from build123d import *

# Parameters (mm, degrees)
SKETCH1_W               = 70
SKETCH1_H               = 80
BOSS_EXTRUDE1_DEPTH     = 21.5
FILLET1_R               = 5
SHELL1_T                = 3
BOSS_EXTRUDE2_REACH     = 59.335
SKETCH3_R               = 5
SPLIT2_SURFACE_1_BACK   = 109.454
SPLIT2_SURFACE_1_DEPTH  = 218.908
SPLIT2_SURFACE_2_BACK   = 109.454
SPLIT2_SURFACE_2_DEPTH  = 218.908
SKETCH4_R               = 1
CUT_EXTRUDE1_DEPTH      = 58.334544561
SKETCH5_R               = 3
CUT_EXTRUDE2_DEPTH      = 7.75
SKETCH6_OUTSIDE_W       = 93.69
SKETCH6_OUTSIDE_H       = 103.69
CUT_EXTRUDE3_DEPTH      = 2
BOSS_EXTRUDE3_START     = 1.7
BOSS_EXTRUDE3_DEPTH     = 1.7
SKETCH8_R               = 5.5
CUT_EXTRUDE4_DEPTH      = 10
SKETCH9_R               = 5
SKETCH9_W               = 20
SKETCH9_H               = 12
CUT_EXTRUDE5_DEPTH      = 10
BOSS_EXTRUDE4_OUTLINE_W = 20
BOSS_EXTRUDE4_OUTLINE_H = 1.5
BOSS_EXTRUDE4_DEPTH     = 7.75
SKETCH12_W              = 29.5
SKETCH12_H              = 12
CUT_EXTRUDE6_DEPTH      = 10
BOSS_EXTRUDE5_DEPTH     = 5


# Read off the part's stored shape, not the designer's step: Boss-Extrude4
with BuildPart() as part:
    # Sketch1 → Boss-Extrude1 (new body)
    with BuildSketch(Plane(origin=(0, 0, 0), x_dir=(1, 0, 0), z_dir=(0, 1, 0))):
        Rectangle(SKETCH1_W, SKETCH1_H)
    extrude(amount=BOSS_EXTRUDE1_DEPTH)

    # Fillet1
    fillet1_edges = [part.edges().sort_by_distance(p)[0] for p in [
        (-35, 10.75, -40),
        (35, 10.75, -40),
        (35, 10.75, 40),
        (-35, 10.75, 40),
    ]]
    fillet(fillet1_edges, radius=FILLET1_R)

    # Shell1 (no face opened: a closed hollow body)
    add(offset(amount=-SHELL1_T, mode=Mode.PRIVATE), mode=Mode.SUBTRACT)

    # Sketch3 → Boss-Extrude2 (add, up to next)
    with BuildSketch(Plane(origin=(0, 21.5, 0), x_dir=(1, 0, 0), z_dir=(0, 1, 0)), mode=Mode.PRIVATE) as boss_extrude2_sk1:
        with Locations((-30, 35)):
            Circle(SKETCH3_R)
    boss_extrude2_tool1 = extrude(boss_extrude2_sk1.sketch, amount=-BOSS_EXTRUDE2_REACH, mode=Mode.PRIVATE) - part.part
    # Sketch3 → Boss-Extrude2 (add, up to next)
    with BuildSketch(Plane(origin=(0, 21.5, 0), x_dir=(1, 0, 0), z_dir=(0, 1, 0)), mode=Mode.PRIVATE) as boss_extrude2_sk2:
        with Locations((30, 35)):
            Circle(SKETCH3_R)
    boss_extrude2_tool2 = extrude(boss_extrude2_sk2.sketch, amount=-BOSS_EXTRUDE2_REACH, mode=Mode.PRIVATE) - part.part
    # Sketch3 → Boss-Extrude2 (add, up to next)
    with BuildSketch(Plane(origin=(0, 21.5, 0), x_dir=(1, 0, 0), z_dir=(0, 1, 0)), mode=Mode.PRIVATE) as boss_extrude2_sk3:
        with Locations((30, -35)):
            Circle(SKETCH3_R)
    boss_extrude2_tool3 = extrude(boss_extrude2_sk3.sketch, amount=-BOSS_EXTRUDE2_REACH, mode=Mode.PRIVATE) - part.part
    # Sketch3 → Boss-Extrude2 (add, up to next)
    with BuildSketch(Plane(origin=(0, 21.5, 0), x_dir=(1, 0, 0), z_dir=(0, 1, 0)), mode=Mode.PRIVATE) as boss_extrude2_sk4:
        with Locations((-30, -35)):
            Circle(SKETCH3_R)
    boss_extrude2_tool4 = extrude(boss_extrude2_sk4.sketch, amount=-BOSS_EXTRUDE2_REACH, mode=Mode.PRIVATE) - part.part
    add(boss_extrude2_tool1.solids().sort_by_distance((-30, 21.5, -35))[0])
    add(boss_extrude2_tool2.solids().sort_by_distance((30, 21.5, -35))[0])
    add(boss_extrude2_tool3.solids().sort_by_distance((30, 21.5, 35))[0])
    add(boss_extrude2_tool4.solids().sort_by_distance((-30, 21.5, 35))[0])


with BuildPart() as body_2:
    # Split2: the piece behind the surface
    add(part.part)
    # Split2 surface: a surface, the sketch's curves swept straight by 218.908 mm
    with BuildLine(Plane(origin=(0, 0, 0), x_dir=(0, 0, -1), z_dir=(1, 0, 0)).offset(-SPLIT2_SURFACE_1_BACK), mode=Mode.PRIVATE) as split2_surface_1_path:
        Line((-40, 10.75), (51.562362236, 10.75))
    split2_surface_1 = Shell.extrude(split2_surface_1_path.wire(), (1 * SPLIT2_SURFACE_1_DEPTH, 0 * SPLIT2_SURFACE_1_DEPTH, 0 * SPLIT2_SURFACE_1_DEPTH))
    split(bisect_by=split2_surface_1, keep=Keep.BOTTOM)


with BuildPart() as part_1:
    add(part.part)

    # Split2: split by a surface, the side it looks to stays
    # Split2 surface: a surface, the sketch's curves swept straight by 218.908 mm
    with BuildLine(Plane(origin=(0, 0, 0), x_dir=(0, 0, -1), z_dir=(1, 0, 0)).offset(-SPLIT2_SURFACE_2_BACK), mode=Mode.PRIVATE) as split2_surface_2_path:
        Line((-40, 10.75), (51.562362236, 10.75))
    split2_surface_2 = Shell.extrude(split2_surface_2_path.wire(), (1 * SPLIT2_SURFACE_2_DEPTH, 0 * SPLIT2_SURFACE_2_DEPTH, 0 * SPLIT2_SURFACE_2_DEPTH))
    split(bisect_by=split2_surface_2, keep=Keep.TOP)


with BuildPart() as cut_extrude1_tool:
    # Sketch4 → Cut-Extrude1 (new, through all)
    with BuildSketch(Plane(origin=(0, 21.5, 0), x_dir=(1, 0, 0), z_dir=(0, 1, 0))):
        with Locations(Location((-30, 35, 0), (0, 0, 270))):
            Circle(SKETCH4_R)
        with Locations(Location((30, 35, 0), (0, 0, 270))):
            Circle(SKETCH4_R)
        with Locations(Location((30, -35, 0), (0, 0, 270))):
            Circle(SKETCH4_R)
        with Locations(Location((-30, -35, 0), (0, 0, 270))):
            Circle(SKETCH4_R)
    extrude(amount=-CUT_EXTRUDE1_DEPTH)


with BuildPart() as part_2:
    add(part_1.part)

    # Cut-Extrude1: cut by cut_extrude1_tool
    add(cut_extrude1_tool.part, mode=Mode.SUBTRACT)

    # Sketch5 → Cut-Extrude2 (cut)
    with BuildSketch(Plane(origin=(0, 21.5, 0), x_dir=(1, 0, 0), z_dir=(0, 1, 0))):
        with Locations(Location((-30, 35, 0), (0, 0, 270))):
            Circle(SKETCH5_R)
        with Locations(Location((30, 35, 0), (0, 0, 270))):
            Circle(SKETCH5_R)
        with Locations(Location((30, -35, 0), (0, 0, 270))):
            Circle(SKETCH5_R)
        with Locations(Location((-30, -35, 0), (0, 0, 270))):
            Circle(SKETCH5_R)
    extrude(amount=-CUT_EXTRUDE2_DEPTH, mode=Mode.SUBTRACT)

    # Sketch6 outside → Cut-Extrude3 (cut)
    with BuildSketch(Plane.XZ.offset(-10.75)):
        Rectangle(SKETCH6_OUTSIDE_W, SKETCH6_OUTSIDE_H)
        with BuildLine():
            Line((-30, -38.5), (30, -38.5))
            ThreePointArc((30, -38.5), (32.474873734, -37.474873734), (33.5, -35))
            Line((33.5, -35), (33.5, 35))
            ThreePointArc((33.5, 35), (32.474873734, 37.474873734), (30, 38.5))
            Line((30, 38.5), (-30, 38.5))
            ThreePointArc((-30, 38.5), (-32.474873734, 37.474873734), (-33.5, 35))
            Line((-33.5, 35), (-33.5, -35))
            ThreePointArc((-33.5, -35), (-32.474873734, -37.474873734), (-30, -38.5))
        make_face(mode=Mode.SUBTRACT)
    extrude(amount=-CUT_EXTRUDE3_DEPTH, mode=Mode.SUBTRACT)


with BuildPart() as body_2_1:
    add(body_2.part)

    # Cut-Extrude1: cut by cut_extrude1_tool
    add(cut_extrude1_tool.part, mode=Mode.SUBTRACT)

    # Sketch7 → Boss-Extrude3 (add)
    with BuildSketch(Plane(origin=(0, 10.75, 0), x_dir=(1, 0, 0), z_dir=(0, 1, 0)).offset(BOSS_EXTRUDE3_START)):
        with BuildLine():
            Line((-30, 40), (30, 40))
            ThreePointArc((30, 40), (33.535533906, 38.535533906), (35, 35))
            Line((35, 35), (35, -35))
            ThreePointArc((35, -35), (33.535533906, -38.535533906), (30, -40))
            Line((30, -40), (-30, -40))
            ThreePointArc((-30, -40), (-33.535533906, -38.535533906), (-35, -35))
            Line((-35, -35), (-35, 35))
            ThreePointArc((-35, 35), (-33.535533906, 38.535533906), (-30, 40))
        make_face()
        with BuildLine():
            Line((30, 38.7), (-30, 38.7))
            ThreePointArc((-30, 38.7), (-32.61629509, 37.61629509), (-33.7, 35))
            Line((-33.7, 35), (-33.7, -35))
            ThreePointArc((-33.7, -35), (-32.61629509, -37.61629509), (-30, -38.7))
            Line((-30, -38.7), (30, -38.7))
            ThreePointArc((30, -38.7), (32.61629509, -37.61629509), (33.7, -35))
            Line((33.7, -35), (33.7, 35))
            ThreePointArc((33.7, 35), (32.61629509, 37.61629509), (30, 38.7))
        make_face(mode=Mode.SUBTRACT)
    extrude(amount=-BOSS_EXTRUDE3_DEPTH)


with BuildPart() as cut_extrude4_tool:
    # Sketch8 → Cut-Extrude4 (new body)
    with BuildSketch(Plane.ZY.offset(35)):
        with Locations((-20, 11.95)):
            Circle(SKETCH8_R)
    extrude(amount=-CUT_EXTRUDE4_DEPTH)


with BuildPart() as part_3:
    add(part_2.part)

    # Cut-Extrude4: cut by cut_extrude4_tool
    add(cut_extrude4_tool.part, mode=Mode.SUBTRACT)


with BuildPart() as body_2_2:
    add(body_2_1.part)

    # Cut-Extrude4: cut by cut_extrude4_tool
    add(cut_extrude4_tool.part, mode=Mode.SUBTRACT)


with BuildPart() as cut_extrude5_tool:
    # Sketch9 → Cut-Extrude5 (new body)
    with BuildSketch(Plane.XY.offset(40)):
        with Locations((16, 11.95)):
            Circle(SKETCH9_R)
        with Locations((-10, 10.75)):
            Rectangle(SKETCH9_W, SKETCH9_H)
    extrude(amount=-CUT_EXTRUDE5_DEPTH)


with BuildPart() as part_4:
    add(part_3.part)

    # Cut-Extrude5: cut by cut_extrude5_tool
    add(cut_extrude5_tool.part, mode=Mode.SUBTRACT)

    # Boss-Extrude4 outline → Boss-Extrude4 (add)
    with BuildSketch(Plane.XZ.offset(-18.5)):
        Polygon((10.5, 37), (7.5, 37), (7.5, 35), (6, 35), (6, 32), (10.5, 32), align=None)
        with Locations((-10, 37.75)):
            Rectangle(BOSS_EXTRUDE4_OUTLINE_W, BOSS_EXTRUDE4_OUTLINE_H)
        with BuildLine():
            Line((-23.5, 35), (-25, 35))
            ThreePointArc((-25, 35), (-25.25658351, 33.41886117), (-26, 32))
            Line((-26, 32), (-23.5, 32))
            Line((-23.5, 32), (-23.5, 35))
        make_face()
        with BuildLine():
            Line((-25, 35), (-25, 37))
            Line((-25, 37), (-25.417424305, 37))
            ThreePointArc((-25.417424305, 37), (-25.105468435, 36.021548218), (-25, 35))
        make_face()
        with BuildLine():
            Line((-28, 37.236067977), (-28, 32.763932023))
            ThreePointArc((-28, 32.763932023), (-27, 35), (-28, 37.236067977))
        make_face()
    extrude(amount=BOSS_EXTRUDE4_DEPTH)


with BuildPart() as body_2_3:
    add(body_2_2.part)

    # Cut-Extrude5: cut by cut_extrude5_tool
    add(cut_extrude5_tool.part, mode=Mode.SUBTRACT)


with BuildPart() as cut_extrude6_tool:
    # Sketch12 → Cut-Extrude6 (new body)
    with BuildSketch(Plane(origin=(0, 0, 37), x_dir=(-1, 0, 0), z_dir=(0, 0, -1))):
        with Locations((8.75, 10.75)):
            Rectangle(SKETCH12_W, SKETCH12_H)
    extrude(amount=-CUT_EXTRUDE6_DEPTH)


with BuildPart() as part_5:
    add(part_4.part)

    # Cut-Extrude6: cut by cut_extrude6_tool
    add(cut_extrude6_tool.part, mode=Mode.SUBTRACT)

    # Sketch14 → Boss-Extrude5 (add)
    with BuildSketch(Plane.XZ.offset(-10.75)):
        Polygon((10.5, 36.8), (7.5, 36.8), (7.5, 35), (6, 35), (6, 32), (10.5, 32), align=None)
    extrude(amount=BOSS_EXTRUDE5_DEPTH)


with BuildPart() as body_2_4:
    add(body_2_3.part)

    # Cut-Extrude6: cut by cut_extrude6_tool
    add(cut_extrude6_tool.part, mode=Mode.SUBTRACT)


solid = body_2_4.part
Verification items for the finished model (mm, model axes). A direction names the side the tool comes from. Give positions to 0.01 mm unless a question says otherwise; leave off trailing zeros. Loops run counter-clockwise (first coordinate to the right, second up) from the corner with the lowest first, then second, coordinate; pieces in that order, holes last. Notation, with made-up numbers: (55, -4.75) - (62, -4.75) arc R11 ccw to (62, 11.25) - close; hole circle Ø7 at (48.5, 18.5). An arc over 180 degrees is marked (long way). Write each question's results on one line, items separated by ' | '.
1) Sectioned sample at A-A on y = 8. Count the separate pieces of the cut face and the enclosed holes in it, plus the area to 3 significant figures.
Solution:
separate pieces: 3 | enclosed holes: 4 | area: 872 mm2
2) Material ranges on L1, parallel to X at y = 5.75, z = -35; L2, parallel to X at y = 4.25, z = -17; L3, parallel to Z at x = -1, y = 3.5, recorded low to high. Write a range as from..to.
Solution:
L1: -35..-31, -29..-25, 25..29, 31..35 | L2: -35..-32, 32..35 | L3: -40..-37, 37..40
3) Mould release check, pull along X, two halves, no side actions. Record for faces 1 (the flat face through (35, 6, 0)), 2 (the flat face through (32.3, 10.75, -14.2)), 3 (the flat face through (34, 12.45, -18)): pulls with the +X half, pulls with the -X half, needs draft (parallel to the pull), parting line crosses it, or undercut.
Solution:
face 1: pulls with the +X half | face 2: undercut | face 3: needs draft
4) Sectioned sample at B-B on x = 27. Record the boundary of the cut face in (y, z).
Solution:
outline: (0, -40) - (12.45, -40) - (12.45, -38.7) - (10.75, -38.7) - (10.75, -31) - (3, -31) - (3, 31) - (10.75, 31) - (10.75, 38.7) - (12.45, 38.7) - (12.45, 40) - (0, 40) - close
5) Tool access check on faces 4 (the flat face through (-9, 4.75, 38)), 5 (the flat face through (0, 7, -37)), 6 (the cylindrical face through (30.84, 5.45, -34.46)). Record the directions out of +Z, -Z, +X, -X, +Y, -Y that give a thin tool (end or side, any length) a straight path to the whole face; none if there is none.
Solution:
face 4: +Z, +Y | face 5: +Y | face 6: +Y, -Y
6) Depth check by flat-ended pin: P1, Ø8, axis at x = -10, z = 12, coming from the +Y side; P2, Ø2.5, axis at x = -30, z = -35, coming from the +Y side; P3, Ø4, axis at x = 6.5, z = -31, coming from the -Y side; P4, Ø1.5, axis at x = -2, z = 39, coming from the +Y side. Enter the tip coordinate at first touch or a pass-through.
Solution:
P1: y = 3 | P2: y = 10.75 | P3: y = 0 | P4: y = 4.75
7) Sectioned sample at C-C on z = -12. Record the boundary of the cut face in (x, y).
Solution:
outline: (-35, 0) - (35, 0) - (35, 12.45) - (33.7, 12.45) - (33.7, 10.75) - (32, 10.75) - (32, 3) - (-32, 3) - (-32, 10.75) - (-33.7, 10.75) - (-33.7, 12.45) - (-35, 12.45) - close
8) Sectioned sample at D-D on x = 16. Record the boundary of the cut face in (y, z), plus the area to 3 significant figures.
Solution:
outline: (0, -40) - (12.45, -40) - (12.45, -38.7) - (10.75, -38.7) - (10.75, -37) - (3, -37) - (3, 37) - (6.95, 37) - (6.95, 40) - (0, 40) - close | area: 277 mm2
